CAD build for the part. Positions are in the model's coordinates, mm. A direction names the side the tool comes from. Round coordinates to 2 decimals unless told otherwise and drop trailing zeros. Order: outer loops, then holes, each group sorted by start corner. A loop starts at its lowest first (then second) coordinate and runs counter-clockwise, first axis right, second up. Notation, with made-up numbers: M 9.5,28 L 35.5,28 A29 cw 35.5,48 Z; hole C 40.25,13.25 d8. An arc over 180 degrees is marked long. Answer as a JSON object with one key per item and string values. Group by question number.
```python
from build123d import *

# Parameters (mm, degrees)
SKETCH1_W                            = 42
SKETCH1_H                            = 42
BOSS_EXTRUDE1_DEPTH                  = 48
SKETCH2_R                            = 2.5
BOSS_EXTRUDE2_DEPTH                  = 20
SKETCH4_W                            = 1.65
SKETCH4_H                            = 48
TAP_DRILL_FOR_M4X0_7_TAP1_AT_2_COUNT = 2
TAP_DRILL_FOR_M4X0_7_TAP1_AT_2_PITCH = 31
TAP_DRILL_FOR_M4X0_7_TAP1_AT_3_COUNT = 2
TAP_DRILL_FOR_M4X0_7_TAP1_AT_3_PITCH = 43.840620434
TAP_DRILL_FOR_M4X0_7_TAP1_AT_4_COUNT = 2
TAP_DRILL_FOR_M4X0_7_TAP1_AT_4_PITCH = 31
TAP_DRILL_FOR_M4X0_7_TAP1_AT_5_COUNT = 2
TAP_DRILL_FOR_M4X0_7_TAP1_AT_5_PITCH = 21.920310217
SKETCH6_R                            = 11
BOSS_EXTRUDE3_DEPTH                  = 2


with BuildPart() as part:
    # Sketch1 → Boss-Extrude1 (new body)
    with BuildSketch(Plane(origin=(0, 0, 0), x_dir=(1, 0, 0), z_dir=(0, 1, 0))):
        Rectangle(SKETCH1_W, SKETCH1_H)
    extrude(amount=BOSS_EXTRUDE1_DEPTH)

    # Sketch2 → Boss-Extrude2 (add)
    with BuildSketch(Plane(origin=(0, 48, 0), x_dir=(1, 0, 0), z_dir=(0, 1, 0))):
        with Locations(Location((0, 0, 0), (0, 0, 270))):
            Circle(SKETCH2_R)
    extrude(amount=BOSS_EXTRUDE2_DEPTH)

    # Sketch4 → Tap Drill for M4x0.7 Tap1 (revolve, cut)
    with BuildSketch(Plane(origin=(-15.5, 48, -15.5), x_dir=(0, 0, 1), z_dir=(1, 0, 0))):
        with Locations((0.825, 24)):
            Rectangle(SKETCH4_W, SKETCH4_H)
    tap_drill_for_m4x0_7_tap1 = revolve(axis=Axis((-15.5, 54.35, -15.5), (0, -1, 0)), mode=Mode.SUBTRACT)

    # Tap Drill for M4x0.7 Tap1 at 2: Tap Drill for M4x0.7 Tap1 ×2
    with Locations(*[(0, 0, i * TAP_DRILL_FOR_M4X0_7_TAP1_AT_2_PITCH) for i in range(1, TAP_DRILL_FOR_M4X0_7_TAP1_AT_2_COUNT)]):
        add(tap_drill_for_m4x0_7_tap1, mode=Mode.SUBTRACT)

    # Tap Drill for M4x0.7 Tap1 at 3: Tap Drill for M4x0.7 Tap1 ×2
    with Locations(*[Vector(0.7071067811865476, 0, 0.7071067811865475) * (i * TAP_DRILL_FOR_M4X0_7_TAP1_AT_3_PITCH) for i in range(1, TAP_DRILL_FOR_M4X0_7_TAP1_AT_3_COUNT)]):
        add(tap_drill_for_m4x0_7_tap1, mode=Mode.SUBTRACT)

    # Tap Drill for M4x0.7 Tap1 at 4: Tap Drill for M4x0.7 Tap1 ×2
    with Locations(*[(i * TAP_DRILL_FOR_M4X0_7_TAP1_AT_4_PITCH, 0, 0) for i in range(1, TAP_DRILL_FOR_M4X0_7_TAP1_AT_4_COUNT)]):
        add(tap_drill_for_m4x0_7_tap1, mode=Mode.SUBTRACT)

    # Tap Drill for M4x0.7 Tap1 at 5: Tap Drill for M4x0.7 Tap1 ×2
    with Locations(*[Vector(0.7071067811865477, 0, 0.7071067811865475) * (i * TAP_DRILL_FOR_M4X0_7_TAP1_AT_5_PITCH) for i in range(1, TAP_DRILL_FOR_M4X0_7_TAP1_AT_5_COUNT)]):
        add(tap_drill_for_m4x0_7_tap1, mode=Mode.SUBTRACT)

    # Sketch6 → Boss-Extrude3 (add)
    with BuildSketch(Plane(origin=(0, 48, 0), x_dir=(1, 0, 0), z_dir=(0, 1, 0))):
        with Locations(Location((0, 0, 0), (0, 0, 270))):
            Circle(SKETCH6_R)
    extrude(amount=BOSS_EXTRUDE3_DEPTH)


solid = part.part
```
Item 1: Cut at D-D, the plane z = 0. Give the cut face in (x, y).
Item 2: Flat gauge pins, fed straight in: pin 1 Ø4 at (y, z) = (56, 0) entering from -X; pin 2 Ø2 at (y, z) = (52.5, 11.5) entering from -X; pin 3 Ø3 at (x, z) = (5.5, 2.5) entering from +Y. Where does each tip first touch, or does it go through?
Item 3: Drill centre lines: line 1 (Z direction, x = -15.5, y = 17); line 2 (X direction, y = 19.5, z = 0). Where is each one in solid material? Low to high. Write a range as [from, to].
Item 4: Two-plate mould, pull along X, no slides. Class faces 1 (the face through (15.004, 23.664, -13.926)), 2 (the face through (-10, 48, -10)), 3 (the face through (-14.868, 23.664, -13.976)), 4 (the face through (-10.74, 48.99, -2.38)): +X half, -X half, draft (parallel to the pull), parting line (faces both ways), or undercut.
Item 5: Cut at B-B, the plane x = -15.5. Give the cut face in (y, z).
Item 6: Cut at C-C, the plane y = 5.5. Give the cut face in (x, z), and give its area (3 significant figures).
Item 7: 3-axis set-ups, long thin cutter, end or side, ignore diameter. For faces 5 (the face through (1.464, 23.664, 0.761)), 6 (the face through (-2.44, 58.87, -0.54)), 7 (the face through (0, 24, 21)): which of +Z, -Z, +X, -X, +Y, -Y reach the whole face in a straight line?
Item 8: Cut at A-A, the plane z = 15.5. Give the cut face in (x, y), and give its area (3 significant figures).
Response values:
{
 "1": {"outline": "M -21,0 L -1.65,0 L -1.65,48 L 1.65,48 L 1.65,0 L 21,0 L 21,48 L 11,48 L 11,50 L 2.5,50 L 2.5,68 L -2.5,68 L -2.5,50 L -11,50 L -11,48 L -21,48 Z"},
 "2": {"pin 1": "x = -2.5", "pin 2": "through", "pin 3": "y = 50"},
 "3": {"line 1": "[-21, -17.15], [-13.85, 13.85], [17.15, 21]", "line 2": "[-21, -1.65], [1.65, 21]"},
 "4": {"face 1": "undercut", "face 2": "draft", "face 3": "undercut", "face 4": "parting line"},
 "5": {"outline": "M 0,-21 L 48,-21 L 48,-17.15 L 0,-17.15 Z; M 0,-13.85 L 48,-13.85 L 48,13.85 L 0,13.85 Z; M 0,17.15 L 48,17.15 L 48,21 L 0,21 Z"},
 "6": {"outline": "M -21,-21 L 21,-21 L 21,21 L -21,21 Z; hole C -15.5,-15.5 d3.3; hole C -15.5,15.5 d3.3; hole C 0,0 d3.3; hole C 15.5,-15.5 d3.3; hole C 15.5,15.5 d3.3", "area": "1,720 mm^2"},
 "7": {"face 5": "-Y", "face 6": "+Y", "face 7": "+Z, +X, -X, +Y, -Y"},
 "8": {"outline": "M -21,0 L -17.15,0 L -17.15,48 L -21,48 Z; M -13.85,0 L 13.85,0 L 13.85,48 L -13.85,48 Z; M 17.15,0 L 21,0 L 21,48 L 17.15,48 Z", "area": "1,700 mm^2"}
}
